```python
from build123d import *

# Parameters (mm, degrees)
SKETCH_1_W           = 380
SKETCH_1_H           = 245
EXTRUDE_1_DEPTH      = 65
EXTRUDE_1_DEPTH_BACK = 65
SKETCH_2_W           = 40
SKETCH_2_H           = 20
EXTRUDE_2_DEPTH      = 25.5
SKETCH_3_W           = 40
SKETCH_3_H           = 60
EXTRUDE_3_DEPTH      = 20
SKETCH_4_R           = 8.5
CUT_EXTRUDE_1_DEPTH  = 296


with BuildPart() as part:
    # Эскиз1 → Бобышка-Вытянуть1 (new body, two sides)
    with BuildSketch(Plane(origin=(0, 0, 0), x_dir=(0, 0, -1), z_dir=(1, 0, 0))) as extrude_1_sk:
        Rectangle(SKETCH_1_W, SKETCH_1_H)
    extrude(amount=EXTRUDE_1_DEPTH)
    extrude(extrude_1_sk.sketch, amount=-EXTRUDE_1_DEPTH_BACK)

    # Эскиз2 → Бобышка-Вытянуть2 (add)
    with BuildSketch(Plane(origin=(0, -122.5, -67.5), x_dir=(-1, 0, 0), z_dir=(0, 1, 0))):
        with Locations((0, -112.5)):
            Rectangle(SKETCH_2_W, SKETCH_2_H)
    extrude_2 = extrude(amount=-EXTRUDE_2_DEPTH)

    # Эскиз3 → Бобышка-Вытянуть3 (add)
    with BuildSketch(Plane(origin=(0, 67.5, -190), x_dir=(1, 0, 0), z_dir=(0, 0, 1))):
        with Locations((0, -185.5)):
            Rectangle(SKETCH_3_W, SKETCH_3_H)
    extrude_3 = extrude(amount=-EXTRUDE_3_DEPTH)

    # Зеркальное отражение1: Бобышка-Вытянуть2, Бобышка-Вытянуть3 across plane
    add(extrude_2.mirror(Plane.ZX))
    add(extrude_3.mirror(Plane.ZX))

    # Эскиз4 → Вырез-Вытянуть1 (cut)
    with BuildSketch(Plane(origin=(0, -148, 0), x_dir=(-1, 0, 0), z_dir=(0, -1, 0))):
        with Locations((0, 190)):
            Circle(SKETCH_4_R)
    extrude(amount=-CUT_EXTRUDE_1_DEPTH, mode=Mode.SUBTRACT)


solid = part.part
```
CAD build for the part. Positions are in the model's coordinates, mm. A direction names the side the tool comes from. Coordinates: 2 decimals unless noted, no trailing zeros. Loops run counter-clockwise (first coordinate to the right, second up) from the corner with the lowest first, then second, coordinate; pieces in that order, holes last. Notation, with made-up numbers: (-20.75, 38) - (18.25, 38) arc R33 cw to (18.25, 72) - close; hole circle Ø8 at (60, 63). An arc over 180 degrees is marked (long way). Use CSV: the item, a comma, the result in double quotes. Start each with the question number.
Q1. Cut at B-B, the plane y = -34. List the corners of the cut face in (x, z).
Q2. Drop flat-ended pins along their axis: P1, Ø8, axis at x = 23.5, y = 53.5, coming from the -Z side; P2, Ø20, axis at y = 126.5, z = -197, coming from the +X side; P3, Ø12, axis at y = 113.5, z = -199.5, coming from the -X side; P4, Ø4, axis at x = -35.5, z = -39, coming from the -Y side. Give the stop position or say it passes through.
Q3. 3-axis set-ups, long thin cutter, end or side, ignore diameter. For faces 1 (the flat face through (0, -148, -181)), 2 (the flat face through (0, -88, -200)), 3 (the flat face through (0, -135, -170)), 4 (the flat face through (65, 2, 3)), 5 (the flat face through (0, 135, -170)): which of +Z, -Z, +X, -X, +Y, -Y reach the whole face in a straight line?
Q4. Two-plate mould, pull along Y, no slides. Class faces 6 (the flat face through (20, -125, -194)), 7 (the flat face through (0, 148, -181)), 8 (the flat face through (-36, -2, -190)): +Y half, -Y half, draft (parallel to the pull), parting line (faces both ways), or undercut.
Q5. Cut at C-C, the plane z = 98. List the corners of the cut face in (x, y), then the cut area to 4 significant figures.
Q6. Probe probe 1 along Y at (x, z) = (-60, 12.5); probe 2 along Z at (x, y) = (42, 22.5); probe 3 along Z at (x, y) = (0, 65). List the from-to ranges inside material, lowest first. Write a range as from..to.
Q7. Cut at A-A, the plane x = 0. List the corners of the cut face in (y, z).
Q8. Cut at D-D, the plane x = 49.5. List the corners of the cut face in (y, z).
Here are the results:
1,outline,"(-65, -190) - (-8.5, -190) arc R8.5 cw to (8.5, -190) - (65, -190) - (65, 190) - (-65, 190) - close"
2,P1,"z = -190"
2,P2,"x = 65"
2,P3,"x = -20"
2,P4,"y = -122.5"
3,face 1,"+Z, -Z, +X, -X, -Y"
3,face 2,"-Z, +X, -X"
3,face 3,"+Z, +X, -X, -Y"
3,face 4,"+Z, -Z, +X, +Y, -Y"
3,face 5,"+Z, +X, -X, +Y"
4,face 6,"draft"
4,face 7,"+Y half"
4,face 8,"undercut"
5,outline,"(-65, -122.5) - (65, -122.5) - (65, 122.5) - (-65, 122.5) - close"
5,area,"31,850 mm2"
6,probe 1,"-122.5..122.5"
6,probe 2,"-190..190"
6,probe 3,"-181.5..190"
7,outline,"(-148, -210) - (-88, -210) - (-88, -198.5) - (-148, -198.5) - close; (-148, -181.5) - (148, -181.5) - (148, -170) - (122.5, -170) - (122.5, 190) - (-122.5, 190) - (-122.5, -170) - (-148, -170) - close; (88, -210) - (148, -210) - (148, -198.5) - (88, -198.5) - close"
8,outline,"(-122.5, -190) - (122.5, -190) - (122.5, 190) - (-122.5, 190) - close"
